Read the model definition and answer for the solid it produces. Units are mm, in the model's axes. Face numbers are marked on the shaded views. Round coordinates to 2 decimals unless told otherwise and drop trailing zeros. Write each loop counter-clockwise with the first axis right and the second up, starting at its lowest first coordinate (ties: lowest second). Pieces come first, ordered by that corner, then holes. Notation, with made-up numbers: (-40, 22.25) -> (-17, 22.25) arc R13 ccw to (-17, 37.25) -> close; hole circle Ø9 at (-27, -25). An arc over 180 degrees is marked (long way). Return JSON: item names as keys, results as strings.
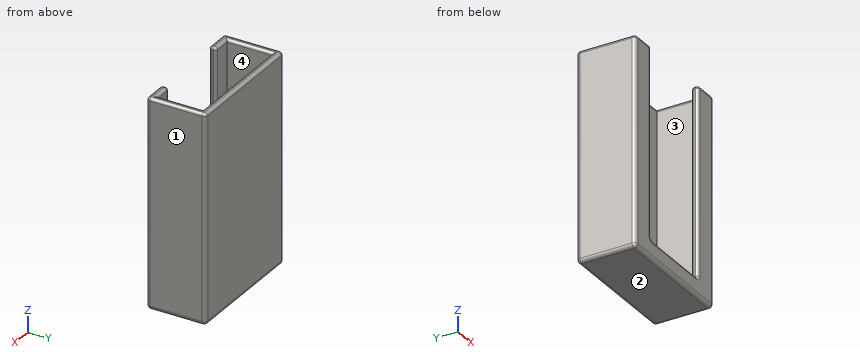
from build123d import *

# Parameters (mm, degrees)
SKETCH_W        = 36
SKETCH_H        = 58
PAD_DEPTH       = 16.5
SKETCH001_W     = 22
SKETCH001_H     = 53
POCKET_DEPTH    = 5
SKETCH002_W     = 32.2
SKETCH002_H     = 12.7
POCKET001_DEPTH = 56
FILLET_R        = 1
FILLET001_R     = 0.75
FILLET002_R     = 0.75


with BuildPart() as part:
    # Sketch → Pad (new body)
    with BuildSketch(Plane.XZ):
        with Locations((18, 29)):
            Rectangle(SKETCH_W, SKETCH_H)
    extrude(amount=PAD_DEPTH)

    # Sketch001 (on Face6 of Pad) → Pocket (cut)
    with BuildSketch(Plane.XZ.offset(16.5)):
        with Locations((18, 31.5)):
            Rectangle(SKETCH001_W, SKETCH001_H)
    extrude(amount=-POCKET_DEPTH, mode=Mode.SUBTRACT)

    # Sketch002 (on Face6 of Pocket) → Pocket001 (cut)
    with BuildSketch(Plane(origin=(0, 0, 58), x_dir=(-1, 0, 0), z_dir=(0, 0, 1))):
        with Locations((-18, 8.25)):
            Rectangle(SKETCH002_W, SKETCH002_H)
    extrude(amount=-POCKET001_DEPTH, mode=Mode.SUBTRACT)

    # Fillet
    fillet_edges = [part.edges().sort_by_distance(p)[0] for p in [
        (36, -16.5, 29),
        (36, 0, 29),
        (36, -8.25, 0),
        (18, -16.5, 0),
        (0, -16.5, 29),
        (0, 0, 29),
        (0, -8.25, 0),
        (18, 0, 0),
    ]]
    fillet(fillet_edges, radius=FILLET_R)

    # Fillet001
    fillet001_edges = [part.edges().sort_by_distance(p)[0] for p in [
        (18, -16.5, 5),
        (7, -15.55, 5),
        (29, -16.5, 31.5),
        (29, -15.55, 5),
        (7, -14.6, 31.5),
        (7, -16.5, 31.5),
        (29, -14.6, 31.5),
        (18, -14.6, 5),
    ]]
    fillet(fillet001_edges, radius=FILLET001_R)

    # Fillet002
    fillet002_edges = [part.edges().sort_by_distance(p)[0] for p in [
        (32.375, -16.5, 58),
        (1.9, -8.25, 58),
        (0.292893, -0.292893, 58),
        (34.1, -8.25, 58),
        (35.707107, -0.292893, 58),
        (18, -1.9, 58),
        (31.925, -14.6, 58),
        (35.707107, -16.207107, 58),
        (29.21967, -14.81967, 58),
        (6.68934, -16.5, 4.68934),
        (29.21967, -16.28033, 58),
        (6.78033, -14.81967, 58),
        (18, 0, 58),
        (0, -8.25, 58),
        (3.625, -16.5, 58),
        (36, -8.25, 58),
    ]]
    fillet(fillet002_edges, radius=FILLET002_R)


solid = part.part
Item 1: For a pull along X with two mould halves and no side action, classify the marked faces 1, 2, 3 and 4 as released by +X, released by -X, zero draft, split by the parting line, or undercut.
Worked answers:
{"face 1": "released by +X", "face 2": "zero draft", "face 3": "undercut", "face 4": "undercut"}
Item 2: Flat-ended cylindrical pins translate along their axes: pin 1 (1.5 mm diameter, centred on x = 24, y = -11, fed in from +Z); pin 2 (6 mm diameter, centred on x = 13, z = 51, fed in from -Y). Find the tip coordinate at first contact, or state that the pin passes through.
Worked answers:
{"pin 1": "stops at z = 2", "pin 2": "stops at y = -1.9"}
Item 3: Section B-B (x = 20) is taken. Give the vertices of the cut face in (y, z), then the cut area to 3 significant figures.
Worked answers:
{"outline": "(-16.5, 1) arc R1 ccw to (-15.5, 0) -> (-1, 0) arc R1 ccw to (0, 1) -> (0, 57.25) arc R0.75 ccw to (-0.75, 58) -> (-1.15, 58) arc R0.75 ccw to (-1.9, 57.25) -> (-1.9, 2) -> (-14.6, 2) -> (-14.6, 4.25) arc R0.75 ccw to (-15.35, 5) -> (-15.75, 5) arc R0.75 ccw to (-16.5, 4.25) -> close", "area": "144 mm2"}
Item 4: Section C-C (y = -6) is taken. Give the vertices of the cut face in (x, z).
Worked answers:
{"outline": "(0, 1) arc R1 ccw to (1, 0) -> (35, 0) arc R1 ccw to (36, 1) -> (36, 57.25) arc R0.75 ccw to (35.25, 58) -> (34.85, 58) arc R0.75 ccw to (34.1, 57.25) -> (34.1, 2) -> (1.9, 2) -> (1.9, 57.25) arc R0.75 ccw to (1.15, 58) -> (0.75, 58) arc R0.75 ccw to (0, 57.25) -> close"}
Item 5: Straight lines are drawn through the part: L1, parallel to X at y = -4.5, z = 55.5; L2, parallel to Y at x = 31.5, z = 53; L3, parallel to Y at x = 22, z = 34. For each, find the intervals that lie inside material, in ascending order. Write a range as [from, to].
Worked answers:
{"L1": "x = [0, 1.9], [34.1, 36]", "L2": "y = [-16.5, -14.6], [-1.9, 0]", "L3": "y = [-1.9, 0]"}
Item 6: Section A-A (z = 19.5) is taken. Give the vertices of the cut face in (x, y), then the cut area to 3 significant figures.
Worked answers:
{"outline": "(0, -15.5) arc R1 ccw to (1, -16.5) -> (6.25, -16.5) arc R0.75 ccw to (7, -15.75) -> (7, -15.35) arc R0.75 ccw to (6.25, -14.6) -> (1.9, -14.6) -> (1.9, -1.9) -> (34.1, -1.9) -> (34.1, -14.6) -> (29.75, -14.6) arc R0.75 ccw to (29, -15.35) -> (29, -15.75) arc R0.75 ccw to (29.75, -16.5) -> (35, -16.5) arc R1 ccw to (36, -15.5) -> (36, -1) arc R1 ccw to (35, 0) -> (1, 0) arc R1 ccw to (0, -1) -> close", "area": "142 mm2"}
